Design review of the part built by this model. Coordinates are the model's own, in mm. A direction names the side the tool comes from. Give positions to 0.01 mm unless a question says otherwise; leave off trailing zeros. Write each loop counter-clockwise with the first axis right and the second up, starting at its lowest first coordinate (ties: lowest second). Pieces come first, ordered by that corner, then holes. Notation, with made-up numbers: (-36, 77) -> (-6, 77) arc R19 ccw to (-6, 108) -> close; hole circle Ø5 at (30.5, 65.25). An arc over 180 degrees is marked (long way). Return JSON: item names as keys, results as strings. Group by question number.
Autodesk Inventor part; units mm, degrees
ref_plane "Work Plane2" through (6.5, 0.5, -10) normal (0, 0, 1) x (1, 0, 0)
ref_plane "Work Plane3" through (6.5, 2, -1.5) normal (0, -1, 0) x (1, 0, 0)
ref_plane "YZ Plane" through (0, 0, 0) normal (1, 0, 0) x (0, 1, 0)
sketch "Sketch1" plane through (0, 0, 0) normal (0, 1, 0) x (-1, 0, 0)
  circle A0 centre (0, 0) radius 4
  line L0 (0, 4) -> (-6.5, 4)
  line L1 (-6.5, 4) -> (-6.5, -4)
  line L2 (-6.5, -4) -> (0, -4)
  line L3 (0, -4) -> (0, 4)
  circle A1 centre (-4.75, 2.75) radius 1.1
  circle A2 centre (-4.75, -2.75) radius 1.1
  point P0 (-6.5, 0)
  dimension "d0" = 8
  dimension "d1" = 6.5
  dimension "d2" = 5.5
  dimension "d3" = 2.75
  dimension "d4" = 1.75
  dimension "d5" = 1.75
  dimension "d6" = 2.2
  dimension "d7" = 2.2
extrude "Extrusion1" add sketch "Sketch1" along normal blind 4
sketch "Sketch2" plane through (6.5, 0, 4) normal (1, 0, 0) x (0, 0, -1)
  line L0 (2.5, 3.5) -> (5.5, 3.5)
  line L1 (5.5, 3.5) -> (5.5, 0.5)
  line L2 (5.5, 0.5) -> (2.5, 0.5)
  line L3 (2.5, 0.5) -> (2.5, 3.5)
  line L4 (0, 4) -> (8, 4)
  line L5 (8, 0) -> (8, 4)
  point P0 (4, 0)
  dimension "d10" = 3
  dimension "d11" = 3
  dimension "d12" = 0.5
  dimension "d13" = 5.5
extrude "Extrusion2" add sketch "Sketch2" along normal blind 4
sketch "Sketch3" plane through (0, 4, 0) normal (0, 1, 0) x (1, 0, 0)
  circle A0 centre (0, 0) radius 2.05
  dimension "d16" = 4.1
extrude "Extrusion3" cut sketch "Sketch3" against normal blind 0.1
sketch "Sketch4" plane through (10.5, 0, 4) normal (1, 0, 0) x (0, 0, -1)
  circle A0 centre (4, 2) radius 1.1
  point P0 (4, 0)
  dimension "d19" = 2.2
ref_plane "Work Plane2" through (6.5, 0.5, -10) normal (0, 0, 1) x (1, 0, 0)
ref_plane "Work Plane1" through (6.5, 0.5, 0) normal (0, 0, 1) x (1, 0, 0)
sketch "Sketch5" plane through (6.5, 0.5, -10) normal (0, 0, 1) x (1, 0, 0)
  circle A0 centre (14, 1.7321) radius 1.1
  line L0 (4, 0) -> (4, 3)
  point P0 (-6.5, -0.5)
  dimension "d23" = 10
  dimension "d24" = 2.2
ref_plane "Work Plane3" through (6.5, 2, -1.5) normal (0, -1, 0) x (1, 0, 0)
sketch "Sketch6" plane through (6.5, 2, -1.5) normal (0, -1, 0) x (1, 0, 0)
  circle A0 centre (4, -8.5) radius 10
  line L0 (4, 3) -> (4, 0)
  point P0 (-6.5, 1.5)
  point P1 (4, 1.5)
  dimension "d25" = 20
  dimension "d26" = 10
revolve "Revolution1" add sketch "Sketch4" angle 90 about axis through (10.5, 0.5, -10) along (0, 1, 0)
equation "\"d5\" = d4"
equation "\"d6\" = d7"
properties part number "CapacitiveSensor"
Q1. Take a section at A-A, the plane x = 4.75. Give the boundary of the cut face in (y, z), plus the area to 3 significant figures.
Q2. Take a section at D-D, the plane x = -0.75. Give the boundary of the cut face in (y, z).
Q3. Take a section at B-B, the plane z = 2.75. Give the boundary of the cut face in (x, y), plus the area to 3 significant figures.
Q4. Take a section at C-C, the plane y = 2.45. Give the boundary of the cut face in (x, z), plus the area to 3 significant figures.
Q5. Mouldability with a two-part tool opening along Z and no side actions: class faces 4 (the face through (3, 2, 4)), 5 (the face through (0, 3.9, 0)), 6 (the face through (8, 2, -1.5)), 7 (the face through (10.5, 3, 1)) as +Z half, -Z half, draft (parallel to the pull), parting line (faces both ways), or undercut.
Q6. Tool access review of faces 1 (the face through (8, 3.5, 0)), 2 (the face through (8, 0.5, 0)), 3 (the face through (3, 2, -4)): name each direction out of +Z, -Z, +X, -X, +Y, -Y from which nothing blocks a thin tool from reaching the whole face with its end or side.
Q7. Insertion check: pin 1 (4.5 mm diameter, centred on x = 0, z = 0, fed in from +Y); pin 2 (2 mm diameter, centred on y = 2.5, z = -4.5, fed in from -X); pin 3 (1 mm diameter, centred on x = 15.5, y = 3, fed in from +Z); pin 4 (2.5 mm diameter, centred on x = 8.5, z = 0, fed in from +Y). Each pin has a flat end and moves straight along its axis. Give the tip position at first contact, or say it passes through.
Q8. For L1, parallel to Z at x = 4.75, y = 2.05; L2, parallel to X at y = 2.3, z = -2; L3, parallel to Z at x = 5.5, y = 0.6, list the stretches that pass through material, from the lowest coordinate up. Write a range as from..to.
Final values:
{
 "1": {"outline": "(0, -4) -> (4, -4) -> (4, -3.85) -> (0, -3.85) -> close; (0, -1.65) -> (4, -1.65) -> (4, 1.65) -> (0, 1.65) -> close; (0, 3.85) -> (4, 3.85) -> (4, 4) -> (0, 4) -> close", "area": "14.4 mm²"},
 "2": {"outline": "(0, -3.93) -> (4, -3.93) -> (4, -1.91) -> (3.9, -1.91) -> (3.9, 1.91) -> (4, 1.91) -> (4, 3.93) -> (0, 3.93) -> close"},
 "3": {"outline": "(-2.9, 0) -> (3.65, 0) -> (3.65, 4) -> (-2.9, 4) -> close; (5.85, 0) -> (6.5, 0) -> (6.5, 4) -> (5.85, 4) -> close", "area": "28.8 mm²"},
 "4": {"outline": "(0, -4) -> (6.5, -4) -> (6.5, -1.5) -> (10.5, -1.5) -> (10.5, -1) arc R9 cw to (19.5, -10) -> (21.5, -10) arc R11 ccw to (10.5, 1) -> (10.5, 1.5) -> (6.5, 1.5) -> (6.5, 4) -> (0, 4) arc R4 ccw to start; hole circle Ø2.2 at (4.75, -2.75); hole circle Ø2.2 at (4.75, 2.75)", "area": "113 mm²"},
 "5": {"face 4": "+Z half", "face 5": "undercut", "face 6": "-Z half", "face 7": "draft"},
 "6": {"face 1": "+Z, -Z, +X, +Y", "face 2": "+Z, -Z, +X, -Y", "face 3": "-Z, -X, +Y, -Y"},
 "7": {"pin 1": "stops at y = 4", "pin 2": "stops at x = -1.94", "pin 3": "stops at z = -0.14", "pin 4": "stops at y = 3.5"},
 "8": {"L1": "z = -4..-3.85, -1.65..1.65, 3.85..4", "L2": "x = -3.46..3.95, 5.55..6.5, 14.49..18.13", "L3": "z = -4..-3.55, -1.95..1.95, 3.55..4"}
}
